Could you check a few things on this drawing? It's one solid part, dimensions in mm from its lowest x, y, z. Give positions to 0.01 mm unless a question says otherwise; leave off trailing zeros. Order: outer loops, then holes, each group sorted by start corner. A loop starts at its lowest first (then second) coordinate and runs counter-clockwise, first axis right, second up. Notation, with made-up numbers: M 17.5,68 L 34.5,68 A23 cw 34.5,102 Z; hole C -8,4 d3. An arc over 180 degrees is marked long. Return JSON: item names as keys, results as strings. Group by question number.
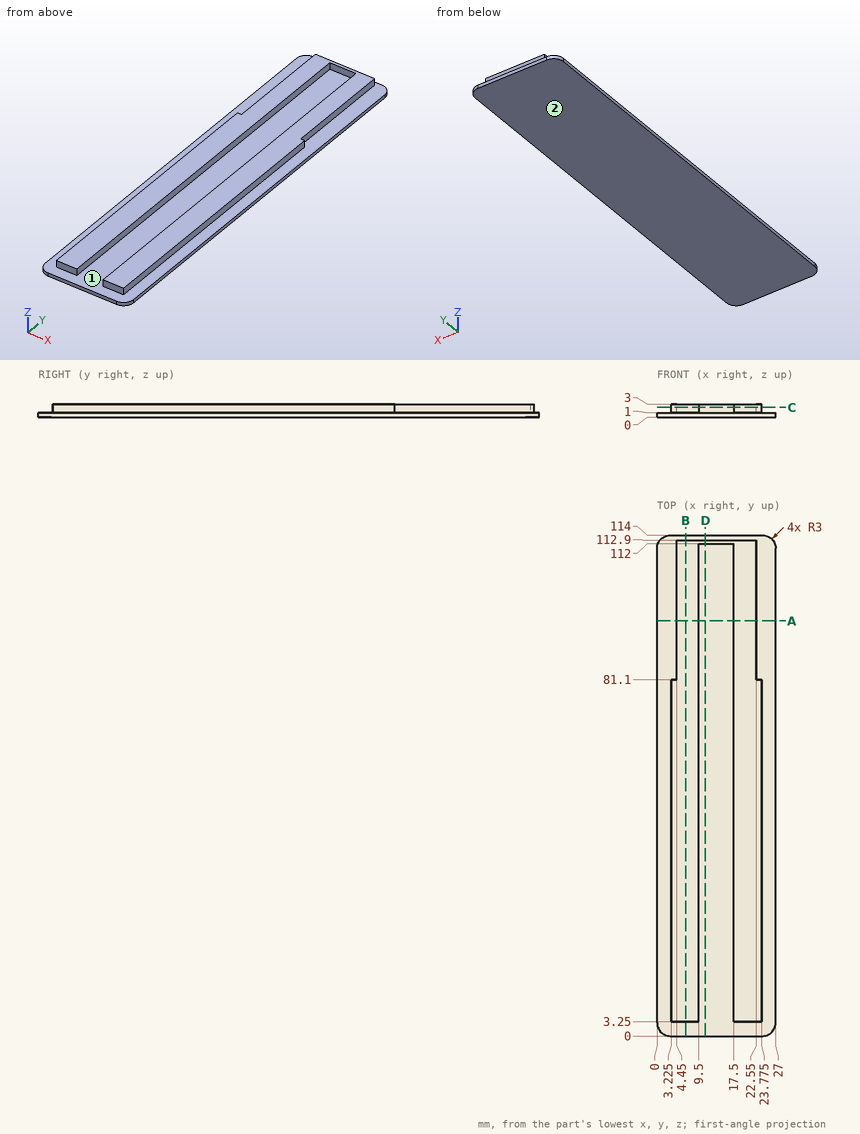
1. Imagine slicing it at A-A, the plane y = 94.5. Please give me the cut outline in (x, z), plus the area to 3 significant figures.
2. Imagine slicing it at B-B, the plane x = 6.5. Please give me the cut outline in (y, z).
3. For pin 1 (0.6 mm diameter, centred on x = 23.5, z = 1.5, fed in from +Y); pin 2 (1 mm diameter, centred on y = 54.5, z = 2, fed in from +X) (3 decimals); pin 3 (0.6 mm diameter, centred on x = 21, z = 2.5, fed in from -Y), each with a flat end and sliding along its axis, tell me the tip position at first contact or that it passes through.
4. I need wall thicknesses on L1, parallel to X at y = 80, z = 2.2 (3 decimals); L2, parallel to X at y = 97.5, z = 2; L3, parallel to Y at x = 21.75, z = 1.9. Which ranges of each line are inside material? Lowest first, please. Write a range as from..to.
5. If we mould it in two halves opening along X, with no side actions, what happens to the marked faces 1 and 2? For each: pulls with the +X half, pulls with the -X half, needs draft (parallel to the pull), parting line crosses it, or undercut.
6. Imagine slicing it at D-D, the plane x = 11. Please give me the cut outline in (y, z), plus the area to 3 significant figures.
7. Imagine slicing it at C-C, the plane z = 2.25. Please give me the cut outline in (x, y) (3 decimals), plus the area to 3 significant figures.
Values:
{
 "1": {"outline": "M 0,0 L 27,0 L 27,1 L 22.55,1 L 22.55,3 L 17.5,3 L 17.5,1 L 9.5,1 L 9.5,3 L 4.45,3 L 4.45,1 L 0,1 Z", "area": "47.2 mm²"},
 "2": {"outline": "M 0,0 L 114,0 L 114,1 L 112.9,1 L 112.9,3 L 3.25,3 L 3.25,1 L 0,1 Z"},
 "3": {"pin 1": "stops at y = 81.1", "pin 2": "stops at x = 23.775", "pin 3": "stops at y = 3.25"},
 "4": {"L1": "x = 3.225..9.5, 17.5..23.775", "L2": "x = 4.45..9.5, 17.5..22.55", "L3": "y = 3.25..112.9"},
 "5": {"face 1": "undercut", "face 2": "needs draft"},
 "6": {"outline": "M 0,0 L 114,0 L 114,1 L 112.9,1 L 112.9,3 L 112,3 L 112,1 L 0,1 Z", "area": "116 mm²"},
 "7": {"outline": "M 3.225,3.25 L 9.5,3.25 L 9.5,112 L 17.5,112 L 17.5,3.25 L 23.775,3.25 L 23.775,81.1 L 22.55,81.1 L 22.55,112.9 L 4.45,112.9 L 4.45,81.1 L 3.225,81.1 Z", "area": "1,310 mm²"}
}
